Autodesk Inventor part; units mm, degrees
ref_plane "YZ Plane" through (0, 0, 0) normal (1, 0, 0) x (0, 1, 0)
ref_plane "XZ Plane" through (0, 0, 0) normal (0, 1, 0) x (-1, 0, 0)
ref_plane "XY Plane" through (0, 0, 0) normal (0, 0, 1) x (1, 0, 0)
sketch "Sketch1" plane through (0, 0, 0) normal (0, 0, 1) x (1, 0, 0)
  line L0 (0, 0) -> (215.9, 0)
  line L1 (215.9, 0) -> (215.9, 25.4)
  line L2 (215.9, 25.4) -> (0, 25.4)
  line L3 (0, 25.4) -> (0, 0)
  dimension "d0" = 215.9
  dimension "d1" = 25.4
extrude "Extrusion1" add sketch "Sketch1" along normal blind 8.89
sketch "Sketch2" plane through (0, 0, 8.89) normal (0, 0, 1) x (1, 0, 0)
  line L0 (0, 0) -> (215.9, 0)
  line L1 (215.9, 25.4) -> (0, 25.4)
  line L2 (0, 25.4) -> (0, 0)
  line L3 (215.9, 25.4) -> (177.8, 25.4)
  line L4 (177.8, 25.4) -> (177.8, 0)
  line L5 (177.8, 0) -> (215.9, 0)
  line L6 (215.9, 0) -> (215.9, 25.4)
  line L7 (177.8, 0) -> (215.9, 0)
  line L8 (215.9, 0) -> (215.9, 12.7)
  line L9 (215.9, 12.7) -> (177.8, 12.7)
  line L10 (177.8, 12.7) -> (177.8, 0)
  line L11 (177.8, 12.7) -> (215.9, 12.7)
  line L12 (215.9, 12.7) -> (215.9, 3.429)
  line L13 (215.9, 3.429) -> (177.8, 3.429)
  line L14 (177.8, 3.429) -> (177.8, 12.7)
  line L15 (177.8, 12.7) -> (215.9, 12.7)
  line L16 (215.9, 12.7) -> (215.9, 21.971)
  line L17 (215.9, 21.971) -> (177.8, 21.971)
  line L18 (177.8, 21.971) -> (177.8, 12.7)
  line L19 (215.9, 25.4) -> (177.8, 25.4)
  line L20 (177.8, 25.4) -> (177.8, 21.971)
  line L21 (177.8, 21.971) -> (215.9, 21.971)
  line L22 (215.9, 21.971) -> (215.9, 25.4)
  dimension "d4" = 38.1
  dimension "d5" = 9.271
  dimension "d6" = 9.271
extrude "Extrusion2" add sketch "Sketch2" along normal blind 8.89 contours L4 L13 L6 L0
sketch "Sketch3" plane through (0, 0, 8.89) normal (0, 0, 1) x (1, 0, 0)
  line L0 (215.9, 25.4) -> (177.8, 25.4)
  line L1 (177.8, 25.4) -> (177.8, 21.9726)
  line L2 (177.8, 21.9726) -> (215.9, 21.9726)
  line L3 (215.9, 21.9726) -> (215.9, 25.4)
extrude "Extrusion3" add sketch "Sketch3" along normal blind 8.89
sketch "Sketch4" plane through (177.8, 3.429, 8.89) normal (0, 1, 0) x (1, 0, 0)
  line L0 (38.1, 0) -> (38.1, -8.89)
  line L1 (0, 0) -> (38.1, 0)
  line L2 (38.1, 0) -> (38.1, -5.08)
  line L3 (38.1, -5.08) -> (0, -5.08)
  line L4 (0, -5.08) -> (0, 0)
  line L5 (38.1, -5.08) -> (0, -5.08)
  line L6 (0, -5.08) -> (0, -8.89)
  line L7 (0, -8.89) -> (38.1, -8.89)
  line L8 (38.1, -8.89) -> (38.1, -5.08)
  point P0 (-177.8, 8.89)
  dimension "d11" = 5.08
extrude "Extrusion4" add sketch "Sketch4" along normal blind 2.54 contours L0 L7 L6 L3
sketch "Sketch5" plane through (177.8, 21.9726, 8.89) normal (0, -1, 0) x (1, 0, 0)
  line L0 (38.1, 0) -> (38.1, 8.89)
  line L1 (0, 0) -> (38.1, 0)
  line L2 (38.1, 0) -> (38.1, 5.08)
  line L3 (38.1, 5.08) -> (0, 5.08)
  line L4 (0, 5.08) -> (0, 0)
  line L5 (0, 5.08) -> (38.1, 5.08)
  line L6 (38.1, 5.08) -> (38.1, 8.89)
  line L7 (38.1, 8.89) -> (0, 8.89)
  line L8 (0, 8.89) -> (0, 5.08)
  point P0 (-177.8, -8.89)
  dimension "d14" = 5.08
extrude "Extrusion5" add sketch "Sketch5" along normal blind 2.54 contours L3 L8 L7 L0
sketch "Sketch6" plane through (215.9, 0, 0) normal (1, 0, 0) x (0, 0, -1)
  line L0 (0, 0) -> (0, 25.4)
  line L1 (0, 25.4) -> (-17.78, 25.4)
  line L2 (-13.97, 19.4326) -> (-17.78, 19.4326)
  line L3 (-13.97, 21.9726) -> (-13.97, 19.4326)
  line L4 (-13.97, 3.429) -> (-13.97, 5.969)
  line L5 (-17.78, 5.969) -> (-13.97, 5.969)
  line L6 (-8.89, 25.4) -> (-5.054, 25.4)
  line L7 (-2.54, 21.9726) -> (-7.62, 21.9726)
  line L8 (-7.62, 21.9726) -> (-7.62, 19.4326)
  line L9 (-2.54, 21.9726) -> (-2.54, 12.7008)
  line L10 (-7.62, 19.4326) -> (-11.43, 19.4326)
  line L11 (-11.43, 19.4326) -> (-11.43, 25.4)
  line L12 (-2.54, 12.7008) -> (-7.9346, 12.7008) construction
  line L13 (-2.54, 3.429) -> (-7.62, 3.429)
  line L14 (-7.62, 3.429) -> (-7.62, 5.969)
  line L15 (-2.54, 3.429) -> (-2.54, 12.7008)
  line L16 (-7.62, 5.969) -> (-11.43, 5.969)
  line L17 (-11.43, 5.969) -> (-11.43, 0.0016)
  line L18 (0, 0) -> (-17.78, 0)
  line L19 (-17.78, 0) -> (-17.78, 25.4)
  line L20 (-17.78, 25.4) -> (0, 25.4)
  line L21 (0, 25.4) -> (0, 0)
  line L22 (-8.89, 19.4326) -> (-8.89, 5.969)
  line L23 (-17.78, 5.969) -> (-13.97, 5.969)
  line L24 (-13.97, 5.969) -> (-13.97, 3.429)
  line L25 (-13.97, 3.429) -> (-11.43, 3.429)
  line L26 (-17.78, 19.4326) -> (-13.97, 19.4326)
  line L27 (-13.97, 19.4326) -> (-13.97, 21.9726)
  line L28 (-13.97, 21.9726) -> (-11.43, 21.9726)
  line L29 (-11.43, 5.969) -> (-7.62, 5.969)
  line L30 (-7.62, 5.969) -> (-7.62, 0)
  line L31 (-7.62, 0) -> (-11.43, 0)
  line L32 (-11.43, 0) -> (-11.43, 5.969)
  dimension "d19" = 3.81
extrude "Extrusion6" add sketch "Sketch6" against normal up to surface (38.1 mm away) contours L18 L30 L13 L15 L9 L7 L8 L10 L11 L1 L0 | L18 L17 L16 L14 L30
extrude "Extrusion7" cut sketch "Sketch6" against normal up to surface (38.1 mm away) contours L18 L19 L5 L4 L25 L17 | L14 L16 L22 L10 L8 L7 L9 L15 L13 | L25 L4 L5 L19 L2 L3 L28 L11 L10 L22 L16 L17 | L11 L28 L3 L2 L19 L1
sketch "Sketch7" plane through (0, 0, 0) normal (0, 0, -1) x (-1, 0, 0)
  line L0 (0, 0) -> (-215.9, 0)
  line L1 (-215.9, 25.4) -> (-177.8, 25.4)
  line L2 (-177.8, 25.4) -> (-177.8, 0)
  line L3 (-177.8, 0) -> (-215.9, 0)
  line L4 (-215.9, 0) -> (-215.9, 25.4)
  circle A0 centre (-196.85, 12.7) radius 4.445
  dimension "d24" = 38.1
  dimension "d25" = 8.89
extrude "Extrusion8" cut sketch "Sketch7" against normal blind 2.54 contours A0
sketch "Sketch8" plane through (0, 0, 8.89) normal (0, 0, 1) x (1, 0, 0)
  circle A0 centre (20.4674, 12.7) radius 6.35
  dimension "d28" = 12.7
extrude "Extrusion9" cut sketch "Sketch8" against normal blind 25.4
properties part number "Piece Two-Diagonal Piece" material "Steel"
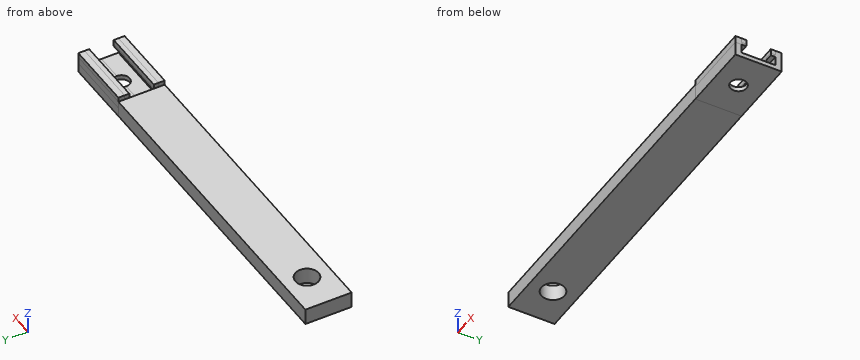
Can you work these out from the model? Positions are in its coordinate system, mm. Give positions to 0.01 mm unless a question says otherwise; leave off trailing zeros. Order: outer loops, then holes, each group sorted by start corner. A loop starts at its lowest first (then second) coordinate and runs counter-clockwise, first axis right, second up. Notation, with made-up numbers: M 11.25,76 L 47.25,76 A25 cw 47.25,106 Z; hole C 17.5,77.5 d6. An arc over 180 degrees is marked long. One line per item, written item: value.
Item 1: If we section it at C-C on x = 154: Write out the boundary of the cut face in (y, z), and give its area (3 significant figures).
Verdict:
outline: M 0,0 L 25.4,0 L 25.4,8.89 L 0,8.89 Z
area: 226 mm2
Item 2: If we section it at A-A on x = 196.85: Write out the boundary of the cut face in (y, z) (3 decimals), and give its area (3 significant figures).
Verdict:
outline: M 0,0 L 8.255,0 L 8.255,2.54 L 3.429,2.54 L 3.429,7.62 L 5.969,7.62 L 5.969,11.43 L 0.002,11.43 Z; M 17.145,0 L 25.4,0 L 25.4,11.43 L 19.433,11.43 L 19.433,7.62 L 21.973,7.62 L 21.973,2.54 L 17.145,2.54 Z
area: 122 mm2
Item 3: Please list where these lines run through material, in increasing order: line 1 (Y direction, x = 196.85, z = 1.5) (3 decimals); line 2 (Y direction, x = 21, z = 5.75); line 3 (Z direction, x = 28, y = 21).
Verdict:
line 1: 0 to 8.255, 17.145 to 25.4
line 2: 0 to 6.37, 19.03 to 25.4
line 3: 0 to 8.89
Item 4: If we section it at B-B on y = 14.5: Write out the boundary of the cut face in (x, z), and give its area (3 significant figures).
Verdict:
outline: M 0,0 L 14.38,0 L 14.38,8.89 L 0,8.89 Z; M 26.56,0 L 192.79,0 L 192.79,2.54 L 177.8,2.54 L 177.8,8.89 L 26.56,8.89 Z; M 200.91,0 L 215.9,0 L 215.9,2.54 L 200.91,2.54 Z
area: 1,550 mm2
Item 5: For pin 1 (4 mm diameter, centred on x = 137.5, z = 9, fed in from +Y); pin 2 (1.3 mm diameter, centred on y = 2.5, z = 10, fed in from -X); pin 3 (1 mm diameter, centred on x = 46, y = 14.5, fed in from +Z); pin 4 (11.5 mm diameter, centred on x = 20.47, y = 12.7, fed in from -Z), each with a flat end and sliding along its axis, tell me the tip position at first contact or that it passes through.
Verdict:
pin 1: y = 25.4
pin 2: x = 177.8
pin 3: z = 8.89
pin 4: through
